Build history of the part. All positions in model axes, mm. A direction names the side the tool comes from. Give positions to 0.01 mm unless a question says otherwise; leave off trailing zeros. Loops run counter-clockwise (first coordinate to the right, second up) from the corner with the lowest first, then second, coordinate; pieces in that order, holes last. Notation, with made-up numbers: M 59.5,17.25 L 113.5,17.25 A20 ccw 113.5,46.25 Z; hole C 1,19 d3. An arc over 180 degrees is marked long. Answer as a JSON object with one key per item and string values. Group by question number.
1. Slice it at D-D (z = -22). List the corners of the cut face in (x, y) (3 decimals).
2. Mould opens along X. For faces 1 (the face through (0, 7, 8.001)), 2 (the face through (-1.121, 7, -7)), 3 (the face through (14.04, -2.25, -23.98)), 4 (the face through (-14.04, -2.25, 23.98)) say: released by +X, released by -X, zero draft, split by the parting line, or undercut.
3. 3-axis set-ups, long thin cutter, end or side, ignore diameter. For faces 5 (the face through (0, 7, -8.001)), 6 (the face through (27.787, -2.254, 0.17)), 7 (the face through (10.3, 0.889, 8.3)): which of +Z, -Z, +X, -X, +Y, -Y reach the whole face in a straight line?
4. Slice it at B-B (y = 16.5). List the corners of the cut face in (x, z), then the cut area to 3 significant figures.
5. Drop flat-ended pins along their axis: pin 1 Ø8 at (y, z) = (1, 12.5) entering from -X; pin 2 Ø0.8 at (y, z) = (11.5, -7) entering from +X; pin 3 Ø0.8 at (y, z) = (13.5, -7) entering from -X; pin 4 Ø3 at (x, z) = (20.62, -11.91) entering from +Y. Give the stop position or say it passes through.
6. Drill centre lines: line 1 along X through (y, z) = (-2, 0); line 2 along Z through (x, y) = (-20.5, -3); line 3 along Y through (x, z) = (23.5, 5.5). Where is each one in solid material? Low to high. Write a range as [from, to].
Autodesk Inventor part; units mm, degrees
ref_plane "Work Plane1" through (0, -2.286, 0) normal (0, 1, 0) x (1, 0, 0)
ref_plane "YZ Plane" through (0, 0, 0) normal (1, 0, 0) x (0, 1, 0)
ref_plane "XZ Plane" through (0, 0, 0) normal (0, 1, 0) x (-1, 0, 0)
sketch "Sketch1" plane through (0, 0, 0) normal (0, 1, 0) x (-1, 0, 0)
  circle A0 centre (0, 0) radius 27.7876
  circle A1 centre (0, 0) radius 23.8125 construction
  line L0 (0, 0) -> (28.7391, -16.5925) construction
  line L1 (0, 0) -> (27.7876, 0) construction
  dimension "d0" = 55.5752
  dimension "d1" = 47.625
  dimension "d2" = 30
extrude "Extrusion1" add sketch "Sketch1" against normal blind 4.572
sketch "Sketch2" plane through (0, 0, 0) normal (0, 1, 0) x (1, 0, 0)
  circle A0 centre (0, 0) radius 23.8125 construction
  line L0 (0, 0) -> (-24.0648, 13.8938) construction
  circle A1 centre (0, 0) radius 27.7876 construction
  line L1 (0, 0) -> (27.7876, 0) construction
  point P0 (-20.6222, 11.9062)
  dimension "d5" = 47.625
  dimension "d6" = 150
hole "Hole1" at (-20.6222, 0, -11.9062) direction (0, -1, 0) diameter 5.1816 end through all
sketch "Sketch3" plane through (0, 0, 0) normal (0, 1, 0) x (1, 0, 0)
  circle A0 centre (-20.6222, 11.9062) radius 2.5908
  line L0 (0, 0) -> (-20.6222, 11.9062) construction
  line L1 (-23.1891, 11.5552) -> (-24.8192, 12.4963)
  line L2 (-21.6016, 14.3048) -> (-23.2317, 15.2459)
  circle A1 centre (0, 0) radius 27.7876
  dimension "d14" = 3.175
  dimension "d15" = 1.5875
extrude "Extrusion2" cut sketch "Sketch3" against normal blind 7.9375 contours A0 L1 A1 L2 picked at (-23.1856, 14.4185)
fillet "Fillet1" radius 0.762 4 edges at (-23.1891, -2.286, -11.5552) (-24.8192, -2.286, -12.4963) (-21.6016, -2.286, -14.3048) (-23.2317, -2.286, -15.2459)
pattern_circular "Circular Pattern1" count 6 over 360 about axis through (0, 0, 0) along (0, -1, 0) of "Hole1", "Extrusion2", "Fillet1"
sketch "Sketch4" plane through (0, 0, 0) normal (0, 1, 0) x (1, 0, 0)
  circle A0 centre (0, 0) radius 14.2875
  dimension "d22" = 28.575
extrude "Extrusion3" add sketch "Sketch4" along normal blind 0.889
chamfer "Chamfer1" distance 0.254 angle 45 1 edges at (-14.2875, 0.889, 0)
fillet "Fillet2" radius 0.254 1 edges at (-14.2875, 0, 0)
ref_plane "Work Plane1" through (0, -2.286, 0) normal (0, 1, 0) x (1, 0, 0)
mirror "Mirror1" about plane through (0, -2.286, 0) normal (0, 1, 0) of "Extrusion3"
chamfer "Chamfer2" distance 0.254 angle 45 1 edges at (-14.2875, -5.461, 0)
fillet "Fillet3" radius 0.254 1 edges at (-14.2875, -4.572, 0)
sketch "Sketch5" plane through (0, 0.889, 0) normal (0, 1, 0) x (1, 0, 0)
  circle A0 centre (0, 0) radius 12.192
  dimension "d33" = 24.384
extrude "Extrusion4" add sketch "Sketch5" along normal blind 19.05
chamfer "Chamfer3" distance 0.254 angle 45 1 edges at (-12.192, 19.939, 0)
chamfer "Chamfer4" distance 0.8128 angle 45 1 edges at (-12.192, 0.889, 0)
sketch "Sketch6" plane through (0, 19.939, 0) normal (0, 1, 0) x (1, 0, 0)
  point P0 (0, 0)
hole "Hole2" at (0, 19.939, 0) direction (0, -1, 0) diameter 12.7 end through all
sketch "Sketch7" plane through (0, 19.939, 0) normal (0, 1, 0) x (1, 0, 0)
  line L0 (-1.1213, 6.2502) -> (-1.1213, 8.001)
  line L1 (1.1375, 6.2473) -> (1.1375, 8.001)
  line L2 (-1.1213, 8.001) -> (1.1375, 8.001)
  circle A0 centre (0, 0) radius 6.35
  dimension "d49" = 8.001
extrude "Extrusion5" cut sketch "Sketch7" against normal through all contours L0 L2 L1 A0
mirror "Mirror2" about plane through (0, 0, 0) normal (0, 0, 1) of "Extrusion5"
fillet "Fillet4" radius 0.127 4 edges at (-1.1213, 7.239, -8.001) (1.1375, 7.239, -8.001) (-1.1213, 7.239, 8.001) (1.1375, 7.239, 8.001)
fillet "Fillet5" radius 0.127 2 edges at (-6.35, 19.939, 0) (6.35, 19.939, 0)
equation "\"d15\" = 0.5 * d14"
properties part number "am-0976" material "Aluminum 6061"
Established:
{
 "1": {"outline": "M -16.975,-4.572 L -1.851,-4.572 L -1.851,0 L -16.975,0 Z; M 1.851,-4.572 L 16.975,-4.572 L 16.975,0 L 1.851,0 Z"},
 "2": {"face 1": "undercut", "face 2": "undercut", "face 3": "released by +X", "face 4": "released by -X"},
 "3": {"face 5": "+Y, -Y", "face 6": "+X, +Y, -Y", "face 7": "+Y"},
 "4": {"outline": "C 0,0 d24.38; hole M -1.12,-7.87 A0.13 ccw -0.99,-8 L 1.01,-8 A0.13 ccw 1.14,-7.87 L 1.14,-6.25 A6.35 ccw 1.14,6.25 L 1.14,7.87 A0.13 ccw 1.01,8 L -0.99,8 A0.13 ccw -1.12,7.87 L -1.12,6.25 A6.35 ccw -1.12,-6.25 Z", "area": "333 mm^2"},
 "5": {"pin 1": "stops at x = -26.41", "pin 2": "stops at x = 10.25", "pin 3": "stops at x = -10.25", "pin 4": "passes through"},
 "6": {"line 1": "x = [-27.79, -6.35], [6.35, 27.79]", "line 2": "z = [-18.76, -14.49], [-9.32, 9.32], [14.49, 18.76]", "line 3": "y = [-4.57, 0]"}
}
